Autodesk Fusion 360 part; units mm, degrees
sketch "Sketch1" plane through (0, 0, 0) normal (0, 0, 1) x (1, 0, 0)
  line L0 (0, 0) -> (40, 0)
  line L1 (40, 0) -> (40, 30)
  line L2 (40, 30) -> (0, 30)
  line L3 (0, 30) -> (0, 0)
  dimension "d1" = 40
  dimension "d2" = 30
extrude "Extrude1" add sketch "Sketch1" along normal blind 5
sketch "Sketch2" plane through (0, 0, 5) normal (0, 0, 1) x (-1, 0, 0)
  line L0 (0, -30) -> (0, 0)
  line L1 (0, 0) -> (-40, 0)
  line L2 (-40, 0) -> (-40, -30)
  line L3 (-40, -30) -> (0, -30)
  line L4 (0, -30) -> (-10, -30)
  line L5 (-10, -30) -> (-10, 0)
  line L6 (-10, 0) -> (0, 0)
  line L7 (0, 0) -> (0, -30)
  dimension "d5" = 10
  dimension "d6" = 30
extrude "Extrude2" add sketch "Sketch2" along normal blind 60 contours L0 L1 L3 L4 L5 L6 L7
sketch "Sketch3" plane through (10, 0, 0) normal (1, 0, 0) x (0, 1, 0)
  line L0 (0, 5) -> (30, 5)
  line L1 (30, 5) -> (30, 65)
  line L2 (30, 65) -> (0, 65)
  line L3 (0, 65) -> (0, 5)
  circle A0 centre (15, 55) radius 7.5
  circle A1 centre (15, 57) radius 7.5
  line L4 (22.5, 55.875) -> (7.5, 55.875)
  line L5 (7.5, 55.875) -> (7.5, 56.125)
  line L6 (7.5, 56.125) -> (22.5, 56.125)
  line L7 (22.5, 56.125) -> (22.5, 55.875)
  line L8 (22.5, 55.875) -> (7.5, 56.125) construction
  line L9 (7.5, 55.875) -> (22.5, 56.125) construction
  point P0 (15, 56)
  dimension "d9" = 15
  dimension "d10" = 15
  dimension "d11" = 15
  dimension "d12" = 0.25
extrude "Extrude3" cut sketch "Sketch3" against normal blind 10 contours A0 L6
sketch "Sketch4" plane through (0, 0, 5) normal (0, 0, 1) x (-1, 0, 0)
  line L0 (-10, -30) -> (-10, 0)
  line L1 (-10, 0) -> (-40, 0)
  line L2 (-40, 0) -> (-40, -30)
  line L3 (-40, -30) -> (-10, -30)
  circle A0 centre (-15, -25) radius 3
  circle A1 centre (-35, -25) radius 3
  circle A2 centre (-15, -5) radius 3
  circle A3 centre (-35, -5) radius 3
  dimension "d17" = 6
  dimension "d18" = 6
  dimension "d19" = 6
  dimension "d20" = 6
extrude "Extrude4" cut sketch "Sketch4" against normal blind 5 contours A0 | A1 | A2 | A3
sketch "Sketch5" plane through (0, 0, 5) normal (0, 0, 1) x (-1, 0, 0)
  circle A0 centre (-15, -25) radius 3
  circle A1 centre (-35, -25) radius 3
  circle A2 centre (-15, -5) radius 3
  circle A3 centre (-35, -5) radius 3
  line L0 (-10, -30) -> (-10, 0)
  line L1 (-10, 0) -> (-40, 0)
  line L2 (-40, 0) -> (-40, -30)
  line L3 (-40, -30) -> (-10, -30)
  circle A4 centre (-15, -5) radius 4.5
  circle A5 centre (-15, -25) radius 4.5
  circle A6 centre (-35, -25) radius 4.5
  circle A7 centre (-35, -5) radius 4.5
  dimension "d23" = 9
  dimension "d24" = 9
  dimension "d25" = 9
  dimension "d26" = 9
extrude "Extrude5" cut sketch "Sketch5" against normal blind 2 contours A4 | A5 | A6 | A7
fillet "Fillet1" radius 1.8 13 edges at (5, 0, 65) (0, 15, 65) (10, 15, 65) (10, 0, 35) (0, 0, 32.5) (25, 0, 5) (40, 0, 2.5) (40, 15, 5) (40, 30, 2.5) (25, 30, 5) (10, 30, 35) (0, 30, 32.5) (5, 30, 65)
Geometry check sheet. Reference: the model listing, model coordinates, mm. A direction names the side the tool comes from. Give positions to 0.01 mm unless a question says otherwise; leave off trailing zeros. Order: outer loops, then holes, each group sorted by start corner. A loop starts at its lowest first (then second) coordinate and runs counter-clockwise, first axis right, second up. Notation, with made-up numbers: (2.5, -36.75) - (57.5, -36.75) arc R5 cw to (57.5, -30.75) - close; hole circle Ø1 at (53, -38). An arc over 180 degrees is marked (long way). Answer in a Markdown table with one row per item. Add a question column.
Q1. Cross-section at A-A, the plane y = 12. Enter the section's corners in (x, z) (3 decimals), then the cut area to 3 significant figures.
Q2. Mould release check, pull along Y, two halves, no side actions. Record for faces 1 (the cylindrical face through (38, 5, 2)), 2 (the cylindrical face through (17.21, 2.97, 1.52)), 3 (the flat face through (24, 15, 5)), 4 (the cylindrical face through (10.45, 0.34, 4.25)): pulls with the +Y half, pulls with the -Y half, needs draft (parallel to the pull), parting line crosses it, or undercut.
Q3. Tool access check on faces 5 (the cylindrical face through (25.096, 0.541, 4.487)), 6 (the flat face through (12, 6, 3)), 7 (the cylindrical face through (39.459, 15.096, 4.487)). Record the directions out of +Z, -Z, +X, -X, +Y, -Y that give a thin tool (end or side, any length) a straight path to the whole face; none if there is none.
Q4. Material ranges on probe 1 along X at (y, z) = (5, 1.9); probe 2 along Y at (x, z) = (35, 2); probe 3 along X at (y, z) = (5, 3.7), recorded low to high. Write a range as from..to.
Q5. Cross-section at C-C, the plane x = 6.5. Enter the section's corners in (y, z) (3 decimals), then the cut area to 3 significant figures.
Q6. Cross-section at B-B, the plane z = 18. Enter the section's corners in (x, y).
Q7. Cross-section at D-D, the plane x = 26.5. Enter the section's corners in (y, z), then the cut area to 3 significant figures.
Q8. Gauge pin test, flat ends, axial feed: pin 1 (5 mm diameter, centred on x = 15, y = 25, fed in from -Z); pin 2 (5 mm diameter, centred on y = 17, z = 48, fed in from +X); pin 3 (10 mm diameter, centred on x = 33.5, y = 26, fed in from +Z); pin 4 (3 mm diameter, centred on x = 10.5, z = 15.5, fed in from -Y). Record the tip position at first contact, or that the pin passes through.
Check values:
| question | item | result |
|---|---|---|
| 1 | outline | (0, 0) - (40, 0) - (40, 3.2) arc R1.8 ccw to (38.2, 5) - (10, 5) - (10, 56.125) - (0, 56.125) - close; (0, 61.874) - (10, 61.874) - (10, 63.2) arc R1.8 ccw to (8.2, 65) - (1.8, 65) arc R1.8 ccw to (0, 63.2) - close |
| 1 | area | 740 mm^2 |
| 2 | face 1 | undercut |
| 2 | face 2 | undercut |
| 2 | face 3 | needs draft |
| 2 | face 4 | pulls with the -Y half |
| 3 | face 5 | +Z, -Y |
| 3 | face 6 | +Z |
| 3 | face 7 | +Z, +X |
| 4 | probe 1 | x = 0..12, 18..32, 38..40 |
| 4 | probe 2 | y = 0..2, 8..22, 28..30 |
| 4 | probe 3 | x = 0..10.5, 19.5..30.5, 39.5..40 |
| 5 | outline | (0, 0) - (30, 0) - (30, 63.2) arc R1.8 ccw to (28.2, 65) - (1.8, 65) arc R1.8 ccw to (0, 63.2) - close; hole (7.585, 56.125) - (22.415, 56.125) arc R7.5 ccw to start |
| 5 | area | 1,880 mm^2 |
| 6 | outline | (0, 1.8) arc R1.8 ccw to (1.8, 0) - (8.2, 0) arc R1.8 ccw to (10, 1.8) - (10, 28.2) arc R1.8 ccw to (8.2, 30) - (1.8, 30) arc R1.8 ccw to (0, 28.2) - close |
| 7 | outline | (0, 0) - (30, 0) - (30, 3.2) arc R1.8 ccw to (28.2, 5) - (1.8, 5) arc R1.8 ccw to (0, 3.2) - close |
| 7 | area | 149 mm^2 |
| 8 | pin 1 | passes through |
| 8 | pin 2 | stops at x = 10 |
| 8 | pin 3 | stops at z = 5 |
| 8 | pin 4 | stops at y = 0.19 |
